Autodesk Inventor part; units mm, degrees
ref_plane "YZ Plane" through (0, 0, 0) normal (1, 0, 0) x (0, 1, 0)
ref_plane "XZ Plane" through (0, 0, 0) normal (0, 1, 0) x (-1, 0, 0)
ref_plane "XY Plane" through (0, 0, 0) normal (0, 0, 1) x (1, 0, 0)
sketch "Sketch1" plane through (0, 0, 0) normal (1, 0, 0) x (0, 1, 0)
  circle A0 centre (0, 0) radius 7.1437
  circle A1 centre (0, 0) radius 19.05
  circle A2 centre (12.7, 0) radius 1.7526
  circle A3 centre (6.35, 10.9985) radius 1.7526
  circle A4 centre (-6.35, 10.9985) radius 1.7526
  circle A5 centre (-12.7, 0) radius 1.7526
  circle A6 centre (-6.35, -10.9985) radius 1.7526
  circle A7 centre (6.35, -10.9985) radius 1.7526
  dimension "d0" = 14.2875
  dimension "d1" = 38.1
  dimension "d4" = 3.5052
  dimension "d5" = 12.7
  dimension "d8" = 360
extrude "Extrusion1" add sketch "Sketch1" along normal blind 1.5875
chamfer "Chamfer1" distance 1.5875 angle 45 6 edges at (0, 10.9474, 0) (0, 4.5974, 10.9985) (0, -14.4526, 0) (0, -8.1026, 10.9985) (0, 4.5974, -10.9985) (0, -8.1026, -10.9985)
properties part number "Spacer 3-8x .125" material "UHMW, Black"
Could you check a few things on this model? Use its own coordinates, in mm. Coordinates: 2 decimals unless noted, no trailing zeros. Loops run counter-clockwise (first coordinate to the right, second up) from the corner with the lowest first, then second, coordinate; pieces in that order, holes last. Notation, with made-up numbers: (40, -31.75) -> (95, -31.75) arc R18 cw to (95, -18.75) -> close; hole circle Ø10 at (79.5, -34.75). An arc over 180 degrees is marked (long way). Answer in a Markdown table with one row per item.
(1) Imagine slicing it at A-A (z = 0). Give the number of separate pieces and of enclosed holes in the cut face, plus the area to 3 significant figures.
Results found:
| item | result |
|---|---|
| separate pieces | 4 |
| enclosed holes | 0 |
| area | 21.6 mm^2 |
(2) Will this pin go through, and if not, where does the flat tip stop? pin 1 Ø4.5 at (y, z) = (6.35, -11) entering from +X.
Results found:
| item | result |
|---|---|
| pin 1 | stops at x = 1.59 |
(3) If I drill on probe 1 along Z at (x, y) = (1.1, 6); probe 2 along Y at (x, z) = (1.1, -2); probe 3 along Y at (x, z) = (0.35, -0.5), over which ranges is the centre line in solid material (lowest first)?
Results found:
| item | result |
|---|---|
| probe 1 | z = -18.08 to -13.21, -8.79 to -3.88, 3.88 to 8.79, 13.21 to 18.08 |
| probe 2 | y = -18.94 to -13.71, -11.69 to -6.86, 6.86 to 11.69, 13.71 to 18.94 |
| probe 3 | y = -19.04 to -15.65, -9.75 to -7.13, 7.13 to 9.75, 15.65 to 19.04 |
(4) Imagine slicing it at D-D (z = -4.5). List the corners of the cut face in (x, y) for me, plus the area to 3 significant figures.
Results found:
| item | result |
|---|---|
| outline | (0, -18.51) -> (1.59, -18.51) -> (1.59, -5.55) -> (0, -5.55) -> close; (0, 5.55) -> (1.59, 5.55) -> (1.59, 18.51) -> (0, 18.51) -> close |
| area | 41.2 mm^2 |
(5) Imagine slicing it at B-B (y = 2.5). List the corners of the cut face in (x, z) for me.
Results found:
| item | result |
|---|---|
| outline | (0, -18.89) -> (1.59, -18.89) -> (1.59, -6.69) -> (0, -6.69) -> close; (0, 6.69) -> (1.59, 6.69) -> (1.59, 18.89) -> (0, 18.89) -> close |
(6) Thinking about a two-plate mould opening in Y: for faces 1 (the face through (0.78, -15.12, 11.59)), 2 (the face through (0.783, 6.814, -2.146)), 3 (the face through (1.588, 8, 0)), which applies, released by +Y, released by -Y, zero draft, split by the parting line, or undercut?
Results found:
| item | result |
|---|---|
| face 1 | split by the parting line |
| face 2 | undercut |
| face 3 | zero draft |
(7) Imagine slicing it at C-C (x = 1.05). List the corners of the cut face in (y, z) for me.
Results found:
| item | result |
|---|---|
| outline | circle Ø38.1 at (0, 0); hole circle Ø4.58 at (-12.7, 0); hole circle Ø4.58 at (-6.35, -11); hole circle Ø4.58 at (-6.35, 11); hole circle Ø14.29 at (0, 0); hole circle Ø4.58 at (6.35, -11); hole circle Ø4.58 at (6.35, 11); hole circle Ø4.58 at (12.7, 0) |
